Build history of the part. All positions in model axes, mm. A direction names the side the tool comes from. Round coordinates to 2 decimals unless told otherwise and drop trailing zeros. Write each loop counter-clockwise with the first axis right and the second up, starting at its lowest first coordinate (ties: lowest second). Pieces come first, ordered by that corner, then holes. Notation, with made-up numbers: (58, 73) -> (85, 73) arc R22 ccw to (85, 84) -> close; hole circle Ø8 at (-2, -17). An arc over 180 degrees is marked (long way). Answer as CSV lines item,"result".
from build123d import *

# Parameters (mm, degrees)
F0_W     = 86.25
F0_H     = 54.25
F1_DEPTH = 5
F2_DEPTH = 1


with BuildPart() as f1:
    # F0 (on Top) → F1 (new body)
    with BuildSketch(Plane.XY):
        with BuildLine():
            ThreePointArc((-43.405657, -24.099012), (-42.673424, -25.866779), (-40.905657, -26.599012))
            Line((-40.905657, -26.599012), (44.094343, -26.599012))
            ThreePointArc((44.094343, -26.599012), (45.86211, -25.866779), (46.594343, -24.099012))
            Line((46.594343, -24.099012), (46.594343, 28.900988))
            ThreePointArc((46.594343, 28.900988), (45.86211, 30.668755), (44.094343, 31.400988))
            Line((44.094343, 31.400988), (-40.905657, 31.400988))
            ThreePointArc((-40.905657, 31.400988), (-42.673424, 30.668755), (-43.405657, 28.900988))
            Line((-43.405657, 28.900988), (-43.405657, -24.099012))
        make_face()
        with Locations((1.538258, 2.464306)):
            Rectangle(F0_W, F0_H, mode=Mode.SUBTRACT)
    extrude(amount=F1_DEPTH)

    # F0 (on Top) → F2 (join)
    with BuildSketch(Plane.XY):
        with Locations((1.538258, 2.464306)):
            Rectangle(F0_W, F0_H)
    extrude(amount=F2_DEPTH)


solid = f1.part
1. Drop flat-ended pins along their axis: pin 1 Ø6 at (x, y) = (-3.5, -4.5) entering from -Z; pin 2 Ø3 at (x, y) = (-22.5, -8) entering from +Z. Give the stop position or say it passes through.
Results found:
pin 1,"stops at z = 0"
pin 2,"stops at z = 1"
2. Cut at B-B, the plane y = 22. Write the cut outline in (x, z), then the cut area to 3 significant figures.
Results found:
outline,"(-43.41, 0) -> (46.59, 0) -> (46.59, 5) -> (44.66, 5) -> (44.66, 1) -> (-41.59, 1) -> (-41.59, 5) -> (-43.41, 5) -> close"
area,"105 mm2"
3. Probe line 1 along Y through (x, z) = (12, 2.5); line 2 along X through (y, z) = (-6, 1.05); line 3 along Z through (x, y) = (-12.5, -8.5). List the from-to ranges inside material, lowest first.
Results found:
line 1,"y = -26.6 to -24.66, 29.59 to 31.4"
line 2,"x = -43.41 to -41.59, 44.66 to 46.59"
line 3,"z = 0 to 1"
4. Cut at C-C, the plane x = 15.5. Write the cut outline in (y, z), then the cut area to 3 significant figures.
Results found:
outline,"(-26.6, 0) -> (31.4, 0) -> (31.4, 5) -> (29.59, 5) -> (29.59, 1) -> (-24.66, 1) -> (-24.66, 5) -> (-26.6, 5) -> close"
area,"73.0 mm2"
5. Which spindle directions (+Z, -Z, +X, -X, +Y, -Y) get a long thin tool onto all of the face, cutting with end or side? Do faces 1 (the cylindrical face through (-42.65, 30.69, 2.46)), 2 (the flat face through (1, 3, 1)). Say none if no direction does.
Results found:
face 1,"+Z, -Z, -X, +Y"
face 2,"+Z"
6. Cut at A-A, the plane z = 2.35. Write the cut outline in (x, y), then the cut area to 3 significant figures.
Results found:
outline,"(-43.41, -24.1) arc R2.5 ccw to (-40.91, -26.6) -> (44.09, -26.6) arc R2.5 ccw to (46.59, -24.1) -> (46.59, 28.9) arc R2.5 ccw to (44.09, 31.4) -> (-40.91, 31.4) arc R2.5 ccw to (-43.41, 28.9) -> close; hole (-41.59, -24.66) -> (44.66, -24.66) -> (44.66, 29.59) -> (-41.59, 29.59) -> close"
area,"536 mm2"
7. Mould opens along Y. For faces 3 (the flat face through (44.663, 2, 3)), 4 (the flat face through (2, 31.401, 2)), 5 (the flat face through (-43.406, 3, 2)) say: +Y half, -Y half, draft (parallel to the pull), parting line (faces both ways), or undercut.
Results found:
face 3,"undercut"
face 4,"+Y half"
face 5,"draft"
